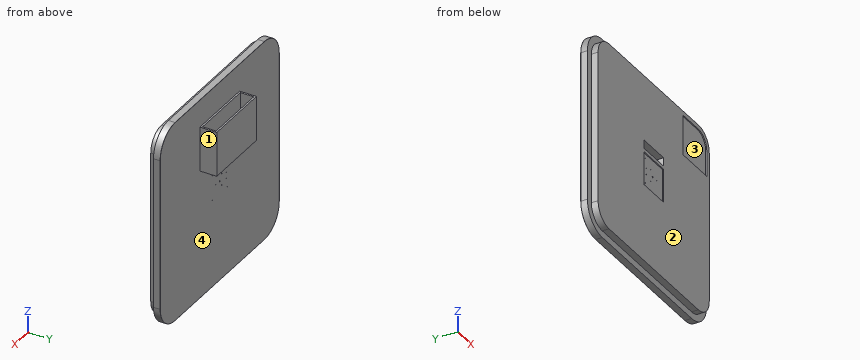
from build123d import *

# Parameters (mm, degrees)
BOSS_EXTRUDE1_DEPTH    = 40
BOSS_EXTRUDE2_DEPTH    = 40
SKETCH3_W              = 200
SKETCH3_H              = 200
CUT_EXTRUDE1_DEPTH     = 6.35
SKETCH4_R              = 2.4892
SKETCH4_R_2            = 3.96875
CUT_EXTRUDE2_DEPTH     = 81
F_10_32_TAPPED_HOLE1_D = 4.0386
SKETCH10_R             = 2.02
SKETCH10_R_2           = 2.032
CUT_EXTRUDE3_DEPTH     = 81
SKETCH11_W             = 200
SKETCH11_H             = 50
CUT_EXTRUDE4_DEPTH     = 81
FILLET1_R              = 1
SKETCH12_W             = 400
SKETCH12_H             = 266
BOSS_EXTRUDE3_DEPTH    = 100
SKETCH13_W             = 380
SKETCH13_H             = 80
CUT_EXTRUDE5_DEPTH     = 266
CUT_EXTRUDE6_DEPTH     = 6.35


with BuildPart() as part:
    # Sketch1 → Boss-Extrude1 (new body)
    with BuildSketch(Plane(origin=(0, 0, 0), x_dir=(1, 0, 0), z_dir=(0, 1, 0))):
        with BuildLine():
            Line((-450, -600), (450, -600))
            ThreePointArc((450, -600), (556.066017178, -556.066017178), (600, -450))
            Line((600, -450), (600, 450))
            ThreePointArc((600, 450), (556.066017178, 556.066017178), (450, 600))
            Line((450, 600), (-450, 600))
            ThreePointArc((-450, 600), (-556.066017178, 556.066017178), (-600, 450))
            Line((-600, 450), (-600, -450))
            ThreePointArc((-600, -450), (-556.066017178, -556.066017178), (-450, -600))
        make_face()
    extrude(amount=BOSS_EXTRUDE1_DEPTH)

    # Sketch2 → Boss-Extrude2 (add)
    with BuildSketch(Plane.XZ):
        with BuildLine():
            Line((560, -450), (560, 450))
            ThreePointArc((560, 450), (527.781745931, 527.781745931), (450, 560))
            Line((450, 560), (-450, 560))
            ThreePointArc((-450, 560), (-527.781745931, 527.781745931), (-560, 450))
            Line((-560, 450), (-560, -450))
            ThreePointArc((-560, -450), (-527.781745931, -527.781745931), (-450, -560))
            Line((-450, -560), (450, -560))
            ThreePointArc((450, -560), (527.781745931, -527.781745931), (560, -450))
        make_face()
    extrude(amount=BOSS_EXTRUDE2_DEPTH)

    # Sketch3 → Cut-Extrude1 (cut)
    with BuildSketch(Plane.XZ.offset(40)):
        Rectangle(SKETCH3_W, SKETCH3_H)
    extrude(amount=-CUT_EXTRUDE1_DEPTH, mode=Mode.SUBTRACT)

    # Sketch4 → Cut-Extrude2 (cut, through all)
    with BuildSketch(Plane(origin=(0, -40, 0), x_dir=(-1, 0, 0), z_dir=(0, -1, 0))):
        with Locations((63.487218193, 19.092554208)):
            Circle(SKETCH4_R)
        with Locations((63.512753284, -19.007437235)):
            Circle(SKETCH4_R)
        Circle(SKETCH4_R_2)
    extrude(amount=-CUT_EXTRUDE2_DEPTH, mode=Mode.SUBTRACT)

    # #10-32 Tapped Hole1 (through all)
    with Locations(Plane(origin=(0, -40, 0), x_dir=(-1, 0, 0), z_dir=(0, -1, 0))):
        with Locations((20.137841448, 34.93381382), (-40.322490944, -0.027024638), (20.184649496, -34.906789182)):
            Hole(F_10_32_TAPPED_HOLE1_D / 2)

    # Sketch10 → Cut-Extrude3 (cut, through all)
    with BuildSketch(Plane(origin=(0, -40, 0), x_dir=(-1, 0, 0), z_dir=(0, -1, 0))):
        with Locations((-74.649981089, 74.549985402)):
            Circle(SKETCH10_R)
        with Locations((74.549274576, 75.710578627)):
            Circle(SKETCH10_R)
        with Locations((74.649981089, -74.549985402)):
            Circle(SKETCH10_R)
        with Locations((-74.549985402, -74.649981089)):
            Circle(SKETCH10_R_2)
    extrude(amount=-CUT_EXTRUDE3_DEPTH, mode=Mode.SUBTRACT)

    # Sketch11 → Cut-Extrude4 (cut, through all)
    with BuildSketch(Plane(origin=(0, -40, 0), x_dir=(-1, 0, 0), z_dir=(0, -1, 0))):
        with Locations((0, -145)):
            Rectangle(SKETCH11_W, SKETCH11_H)
    extrude(amount=-CUT_EXTRUDE4_DEPTH, mode=Mode.SUBTRACT)

    # Fillet1
    fillet1_edges = [part.edges().sort_by_distance(p)[0] for p in [
        (-556.066017178, 40, -556.066017178),
        (-600, 40, 0),
        (-556.066017178, 40, 556.066017178),
        (0, 40, 600),
        (556.066017178, 40, 556.066017178),
        (600, 40, 0),
        (556.066017178, 40, -556.066017178),
        (0, 40, -600),
    ]]
    fillet(fillet1_edges, radius=FILLET1_R)

    # Sketch12 → Boss-Extrude3 (add)
    with BuildSketch(Plane(origin=(0, 40, 0), x_dir=(1, 0, 0), z_dir=(0, 1, 0))):
        with Locations((0, -303)):
            Rectangle(SKETCH12_W, SKETCH12_H)
    extrude(amount=BOSS_EXTRUDE3_DEPTH)

    # Sketch13 → Cut-Extrude5 (cut)
    with BuildSketch(Plane.XY.offset(436)):
        with Locations((0, 90)):
            Rectangle(SKETCH13_W, SKETCH13_H)
    extrude(amount=-CUT_EXTRUDE5_DEPTH, mode=Mode.SUBTRACT)

    # Sketch14 → Cut-Extrude6 (cut)
    with BuildSketch(Plane(origin=(0, -40, 0), x_dir=(-1, 0, 0), z_dir=(0, -1, 0))):
        with BuildLine():
            Line((-450, -535), (-295, -535))
            Line((-295, -535), (-295, -295))
            Line((-295, -295), (-535, -295))
            Line((-535, -295), (-535, -450))
            ThreePointArc((-535, -450), (-510.104076401, -510.104076401), (-450, -535))
        make_face()
    extrude(amount=-CUT_EXTRUDE6_DEPTH, mode=Mode.SUBTRACT)


solid = part.part
Design review of the part built by this model. Coordinates are the model's own, in mm. Face numbers are marked on the shaded views. A direction names the side the tool comes from. Give positions to 0.01 mm unless a question says otherwise; leave off trailing zeros. Order: outer loops, then holes, each group sorted by start corner. A loop starts at its lowest first (then second) coordinate and runs counter-clockwise, first axis right, second up.
1. Mouldability with a two-part tool opening along Z and no side actions: class the marked faces 3 and 4 as +Z half, -Z half, draft (parallel to the pull), parting line (faces both ways), or undercut.
Solution:
face 3: undercut
face 4: draft
2. Add section A-A, the plane y = 101. State the section outline as (x, z) points, then the cut area to 3 significant figures.
Solution:
outline: (-200, 170) - (-190, 170) - (-190, 436) - (-200, 436) - close; (190, 170) - (200, 170) - (200, 436) - (190, 436) - close
area: 5,320 mm2
3. Tool access review of the marked faces 1 and 2: name each direction out of +Z, -Z, +X, -X, +Y, -Y from which nothing blocks a thin tool from reaching the whole face with its end or side.
Solution:
face 1: +Z, -Z, +X, +Y
face 2: +Z, -Z, +X, -X, -Y
4. Add section C-C, the plane x = -264.5. State the section outline as (y, z) points.
Solution:
outline: (-40, -560) - (0, -560) - (0, -600) - (39, -600) arc R1 ccw to (40, -599) - (40, 599) arc R1 ccw to (39, 600) - (0, 600) - (0, 560) - (-40, 560) - close
5. To check wall thickness, follow L1, parallel to X at y = -4, z = 0; L2, parallel to Z at x = 0, y = -10; L3, parallel to Y at x = 250, z = 207. State the ranges of each line that lie inside material, in increasing order.
Solution:
L1: x = -560 to -3.97, 3.97 to 38.3, 42.34 to 560
L2: z = -560 to -3.97, 3.97 to 120, 170 to 560
L3: y = -40 to 40
6. For pin 1 Ø1 at (x, z) = (-308, -84.5) entering from +Y; pin 2 Ø12 at (y, z) = (-22, -85) entering from +X; pin 3 Ø12 at (x, y) = (88.5, -29.5) entering from +Z, all flat-tipped, find the tip position at first contact; note any pin that passes through.
Solution:
pin 1: stops at y = 40
pin 2: stops at x = 560
pin 3: stops at z = 560
7. Add section B-B, the plane z = -311. State the section outline as (x, y) points, then the cut area to 3 significant figures.
Solution:
outline: (-600, 0) - (-560, 0) - (-560, -40) - (560, -40) - (560, 0) - (600, 0) - (600, 39) arc R1 ccw to (599, 40) - (-599, 40) arc R1 ccw to (-600, 39) - close
area: 92,800 mm2
